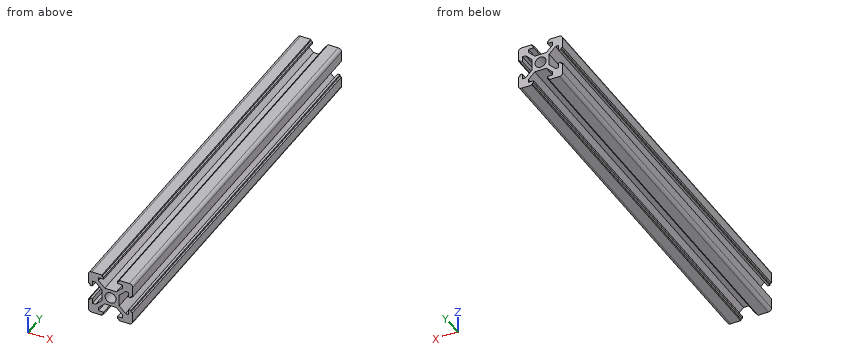
```python
from build123d import *

# Parameters (mm, degrees)
SKETCH1_R           = 2.5
BOSS_EXTRUDE1_DEPTH = 180


with BuildPart() as part:
    # Sketch1 → Boss-Extrude1 (new body)
    with BuildSketch(Plane(origin=(0, 0, 0), x_dir=(1, 0, 0), z_dir=(0, 1, 0))):
        with BuildLine():
            Line((3.9, 10), (8.5, 10))
            ThreePointArc((8.5, 10), (9.560660172, 9.560660172), (10, 8.5))
            Line((10, 8.5), (10, 3.9))
            Line((10, 3.9), (9.2, 3.9))
            Line((9.2, 3.9), (9.2, 3.1))
            Line((9.2, 3.1), (8.2, 3.1))
            Line((8.2, 3.1), (8.2, 5.5))
            Line((8.2, 5.5), (6.77, 5.5))
            Line((6.77, 5.5), (3.9, 2.63))
            Line((3.9, 2.63), (3.9, 0))
            Line((3.9, 0), (3.9, -2.63))
            Line((3.9, -2.63), (6.77, -5.5))
            Line((6.77, -5.5), (8.2, -5.5))
            Line((8.2, -5.5), (8.2, -3.1))
            Line((8.2, -3.1), (9.2, -3.1))
            Line((9.2, -3.1), (9.2, -3.9))
            Line((9.2, -3.9), (10, -3.9))
            Line((10, -3.9), (10, -8.5))
            ThreePointArc((10, -8.5), (9.560660172, -9.560660172), (8.5, -10))
            Line((8.5, -10), (3.9, -10))
            Line((3.9, -10), (3.9, -9.2))
            Line((3.9, -9.2), (3.1, -9.2))
            Line((3.1, -9.2), (3.1, -8.2))
            Line((3.1, -8.2), (5.5, -8.2))
            Line((5.5, -8.2), (5.5, -6.77))
            Line((5.5, -6.77), (2.63, -3.9))
            Line((2.63, -3.9), (0, -3.9))
            Line((0, -3.9), (-2.63, -3.9))
            Line((-2.63, -3.9), (-5.5, -6.77))
            Line((-5.5, -6.77), (-5.5, -8.2))
            Line((-5.5, -8.2), (-3.1, -8.2))
            Line((-3.1, -8.2), (-3.1, -9.2))
            Line((-3.1, -9.2), (-3.9, -9.2))
            Line((-3.9, -9.2), (-3.9, -10))
            Line((-3.9, -10), (-8.5, -10))
            ThreePointArc((-8.5, -10), (-9.560660172, -9.560660172), (-10, -8.5))
            Line((-10, -8.5), (-10, -3.9))
            Line((-10, -3.9), (-9.2, -3.9))
            Line((-9.2, -3.9), (-9.2, -3.1))
            Line((-9.2, -3.1), (-8.2, -3.1))
            Line((-8.2, -3.1), (-8.2, -5.5))
            Line((-8.2, -5.5), (-6.77, -5.5))
            Line((-6.77, -5.5), (-3.9, -2.63))
            Line((-3.9, -2.63), (-3.9, 0))
            Line((-3.9, 0), (-3.9, 2.63))
            Line((-3.9, 2.63), (-6.77, 5.5))
            Line((-6.77, 5.5), (-8.2, 5.5))
            Line((-8.2, 5.5), (-8.2, 3.1))
            Line((-8.2, 3.1), (-9.2, 3.1))
            Line((-9.2, 3.1), (-9.2, 3.9))
            Line((-9.2, 3.9), (-10, 3.9))
            Line((-10, 3.9), (-10, 8.5))
            ThreePointArc((-10, 8.5), (-9.560660172, 9.560660172), (-8.5, 10))
            Line((-8.5, 10), (-3.9, 10))
            Line((-3.9, 10), (-3.9, 9.2))
            Line((-3.9, 9.2), (-3.1, 9.2))
            Line((-3.1, 9.2), (-3.1, 8.2))
            Line((-3.1, 8.2), (-5.5, 8.2))
            Line((-5.5, 8.2), (-5.5, 6.77))
            Line((-5.5, 6.77), (-2.63, 3.9))
            Line((-2.63, 3.9), (2.63, 3.9))
            Line((2.63, 3.9), (5.5, 6.77))
            Line((5.5, 6.77), (5.5, 8.2))
            Line((5.5, 8.2), (3.1, 8.2))
            Line((3.1, 8.2), (3.1, 9.2))
            Line((3.1, 9.2), (3.9, 9.2))
            Line((3.9, 9.2), (3.9, 10))
        make_face()
        Circle(SKETCH1_R, mode=Mode.SUBTRACT)
    extrude(amount=BOSS_EXTRUDE1_DEPTH)


solid = part.part
```
Geometry check sheet. Reference: the model listing, model coordinates, mm. Give positions to 0.01 mm unless a question says otherwise; leave off trailing zeros. Loops run counter-clockwise (first coordinate to the right, second up) from the corner with the lowest first, then second, coordinate; pieces in that order, holes last. Notation, with made-up numbers: M 33,34.25 L 38,34.25 A29 ccw 38,73.25 Z; hole C 21.5,-3.5 d3. An arc over 180 degrees is marked long. Write item = value, one per line.
(1) Gauge pin test, flat ends, axial feed: pin 1 Ø10 at (x, z) = (6, 7) entering from -Y; pin 2 Ø2 at (y, z) = (102, -0.5) entering from +X; pin 3 Ø2.5 at (x, y) = (1.5, 121) entering from +Z; pin 4 Ø4 at (x, y) = (0, 53) entering from -Z. Record the tip position at first contact, or that the pin passes through.
Answer below:
pin_1 = 0
pin_2 = 3.9
pin_3 = 4.02
pin_4 = -3.9
(2) Sectioned sample at B-B, the plane z = 0. Record the cut outline in (x, y), plus the area to 3 significant figures.
Answer below:
outline = M -3.9,0 L -2.5,0 L -2.5,180 L -3.9,180 Z; M 2.5,0 L 3.9,0 L 3.9,180 L 2.5,180 Z
area = 504 mm2
(3) Sectioned sample at A-A, the plane x = 0. Record the cut outline in (y, z), plus the area to 3 significant figures.
Answer below:
outline = M 0,-3.9 L 180,-3.9 L 180,-2.5 L 0,-2.5 Z; M 0,2.5 L 180,2.5 L 180,3.9 L 0,3.9 Z
area = 504 mm2
(4) Material ranges on line 1 (Z direction, x = 0, y = 120.5); line 2 (Z direction, x = -3.5, y = 12), recorded low to high. Write a range as [from, to].
Answer below:
line_1 = [-3.9, -2.5], [2.5, 3.9]
line_2 = [-9.2, -8.2], [-4.77, 4.77], [8.2, 9.2]
